Input: part model. Units: mm. Frame: model coordinates. A direction names the side the tool comes from. Give positions to 0.01 mm unless a question says otherwise; leave off trailing zeros. Loops run counter-clockwise (first coordinate to the right, second up) from the corner with the lowest first, then second, coordinate; pieces in that order, holes last. Notation, with made-up numbers: M 34,58 L 86,58 A21 ccw 86,62 Z; hole C -16,65.5 d11. An arc over 180 degrees is marked long. Return JSON: item names as keys, results as strings. Group by question number.
```python
from build123d import *

# Parameters (mm, degrees)
F1_DEPTH = 15
F2_R     = 12.5
F3_DEPTH = 914.4
F5_DEPTH = 914.4
F7_DEPTH = 15
F9_DEPTH = 914.4


with BuildPart() as f1:
    # F0 (on Front) → F1 (new body)
    with BuildSketch(Plane.XZ):
        Polygon((101.6, 101.6), (0, 0), (0, -304.8), (304.8, -304.8), (304.8, 0), (203.2, 101.6), align=None)
    extrude(amount=F1_DEPTH)

    # F2 (on face) → F3 (join)
    with BuildSketch(Plane.XZ.offset(15)):
        with Locations((152.4, 87.9872098923)):
            Circle(F2_R)
    extrude(amount=F3_DEPTH)

    # F4 (on face) → F5 (join)
    with BuildSketch(Plane.XZ.offset(15)):
        Polygon((294.8, 0), (294.8, -294.8), (10, -294.8), (10, 0), (0, 0), (0, -304.8), (304.8, -304.8), (304.8, 0), align=None)
    extrude(amount=F5_DEPTH)

    # F6 (on face) → F7 (join)
    with BuildSketch(Plane.XZ.offset(929.4)):
        Polygon((0, 0), (0, -304.8), (304.8, -304.8), (304.8, 0), (203.2, 101.6), (101.6, 101.6), align=None)
    extrude(amount=F7_DEPTH)

    # F8 (on face) → F9 (join)
    with BuildSketch(Plane.XZ.offset(15)):
        Polygon((10, -147.4), (152.4, -147.4), (152.4, -118.5992388964), (120, -118.5992388964), (120, -138.5992388964), (10, -138.5992388964), align=None)
    extrude(amount=F9_DEPTH)


solid = f1.part
```
Item 1: Section C-C, the plane y = -522.5. Return loops of the section in (x, z).
Item 2: Pull-direction query (Y, two-part tool) for faces 1 (the face through (150, -944.4, -99)), 2 (the face through (150, -929.4, -94)), 3 (the face through (254.7, -7.4, 50.1)); classes: pulls with the +Y half, pulls with the -Y half, needs draft (parallel to the pull), parting line crosses it, or undercut.
Item 3: Section A-A, the plane z = -17.5. Return loops of the section in (x, y), then the cut area to 3 significant figures.
Item 4: Reachability of faces 4 (the face through (10, -466, -70)), 5 (the face through (52, -937, 52)), 6 (the face through (10, -466, -222)) from +Z, -Z, +X, -X, +Y, -Y: full face, straight path, thin tool, end or side. Return the list, or none.
Item 5: Material intervals for line 1 (Z direction, x = 42, y = -675); line 2 (X direction, y = -48, z = -91); line 3 (Y direction, x = 124.5, z = -218), sorted ascending. Write a range as from..to.
Item 6: Section D-D, the plane x = 182. Return loops of the section in (y, z), then the cut area to 3 significant figures.
Item 7: Section B-B, the plane x = 236. Return loops of the section in (y, z), then the cut area to 3 significant figures.
Item 8: First-contact query: pin 1 Ø3 at (x, y) = (110.5, -475.5) entering from +Z; pin 2 Ø3 at (x, y) = (7, -676) entering from +Z. Flat tips, straight axial feed; report the tip coordinate or a pass-through.
Answer below:
{
 "1": {"outline": "M 0,-304.8 L 304.8,-304.8 L 304.8,0 L 294.8,0 L 294.8,-294.8 L 10,-294.8 L 10,-147.4 L 152.4,-147.4 L 152.4,-118.6 L 120,-118.6 L 120,-138.6 L 10,-138.6 L 10,0 L 0,0 Z; C 152.4,87.99 d25"},
 "2": {"face 1": "pulls with the -Y half", "face 2": "undercut", "face 3": "needs draft"},
 "3": {"outline": "M 0,-944.4 L 304.8,-944.4 L 304.8,0 L 0,0 Z; hole M 10,-929.4 L 294.8,-929.4 L 294.8,-15 L 10,-15 Z", "area": "27,400 mm^2"},
 "4": {"face 4": "+Z", "face 5": "+Z, -X, +Y, -Y", "face 6": "none"},
 "5": {"line 1": "-304.8..-294.8, -147.4..-138.6", "line 2": "0..10, 294.8..304.8", "line 3": "-944.4..-929.4, -15..0"},
 "6": {"outline": "M -944.4,-304.8 L 0,-304.8 L 0,101.6 L -15,101.6 L -15,-294.8 L -929.4,-294.8 L -929.4,101.6 L -944.4,101.6 Z", "area": "21,300 mm^2"},
 "7": {"outline": "M -944.4,-304.8 L 0,-304.8 L 0,68.8 L -15,68.8 L -15,-294.8 L -929.4,-294.8 L -929.4,68.8 L -944.4,68.8 Z", "area": "20,400 mm^2"},
 "8": {"pin 1": "z = -138.6", "pin 2": "z = 0"}
}
